from build123d import *

# Parameters (mm, degrees)
F3_DEPTH = 25.4


with BuildPart() as f1:
    # F0 (on Front) → F1 (revolve)
    with BuildSketch(Plane.XZ):
        Polygon((4.520118, 0), (0, 0), (0, -7.362884), (0, -8.120686), (1.567202, -8.120686), (1.567202, -14.471013), (1.567202, -16.159639), (4.721958, -14.471013), (31.757258, 0), (28.579464, 0), (5.046357, -12.607159), (5.046357, 0), align=None)
    revolve(axis=Axis((0, 0, -4.060343), (0, 0, -1)))

    # F2 (on Top) → F3 (cut)
    with BuildSketch(Plane.XY):
        with BuildLine():
            ThreePointArc((-4.51249, 3.106461), (0, 5.478381), (4.51249, 3.106461))
            Line((4.51249, 3.106461), (28.376638, 3.106461))
            ThreePointArc((28.376638, 3.106461), (0, 28.546168), (-28.376638, 3.106461))
            Line((-28.376638, 3.106461), (-4.51249, 3.106461))
        make_face()
        with BuildLine():
            Line((28.376638, -3.106461), (4.51249, -3.106461))
            ThreePointArc((4.51249, -3.106461), (0, -5.478381), (-4.51249, -3.106461))
            Line((-4.51249, -3.106461), (-28.376638, -3.106461))
            ThreePointArc((-28.376638, -3.106461), (0, -28.546168), (28.376638, -3.106461))
        make_face()
    extrude(amount=-F3_DEPTH, mode=Mode.SUBTRACT)


solid = f1.part
Geometry check sheet. Reference: the model listing, model coordinates, mm. A direction names the side the tool comes from. Coordinates: 2 decimals unless noted, no trailing zeros. Order: outer loops, then holes, each group sorted by start corner. A loop starts at its lowest first (then second) coordinate and runs counter-clockwise, first axis right, second up. Notation, with made-up numbers: (-18, -19.5) -> (16, -19.5) arc R32 ccw to (16, 17.5) -> close; hole circle Ø8 at (4, 38). An arc over 180 degrees is marked (long way). Use a Markdown table: item, result. Add a question column.
1. Mould release check, pull along Y, two halves, no side actions. Record for faces 4 (the face through (-0.074, 5.478, -13.209)), 5 (the face through (5.4, -0.6, -12.4)), 6 (the face through (0, 0, 0)): pulls with the +Y half, pulls with the -Y half, needs draft (parallel to the pull), parting line crosses it, or undercut.
2. Cross-section at C-C (x = -0.5). Give the number of separate pieces and of enclosed holes in the cut face, and give its area (3 significant figures).
3. Go/stop test with flat-tipped pins: pin 1 Ø4 at (x, z) = (22, -5) entering from +Y; pin 2 Ø2 at (x, y) = (2.5, 1) entering from -Z; pin 3 Ø4 at (x, z) = (-17.5, -8) entering from -Y; pin 4 Ø1 at (x, y) = (-11.5, -5) entering from -Z. Record where each tip stops, or that it passes through.
4. Set-up check for faces 1 (the face through (0.58, 28.54, -0.86)), 2 (the face through (2.713, -4.255, -6.215)), 3 (the face through (-0.204, -1.554, -12.196)): record each of +Z, -Z, +X, -X, +Y, -Y from which the full face is reachable in a straight line by a thin tool's end or side.
5. Cross-section at B-B (z = -2.75). Enter the section's corners in (x, y).
6. Cross-section at A-A (z = -11.5). Enter the section's corners in (x, y).
7. Material ranges on L1, parallel to Y at x = 0, z = -14; L2, parallel to Y at x = 0, z = -12.25; L3, parallel to X at y = 0.5, z = -5.25, recorded low to high.
Filled sheet:
| question | item | result |
|---|---|---|
| 1 | face 4 | pulls with the +Y half |
| 1 | face 5 | undercut |
| 1 | face 6 | needs draft |
| 2 | separate pieces | 3 |
| 2 | enclosed holes | 0 |
| 2 | area | 139 mm2 |
| 3 | pin 1 | y = 3.11 |
| 3 | pin 2 | z = -16.09 |
| 3 | pin 3 | y = -3.11 |
| 3 | pin 4 | through |
| 4 | face 1 | +Z, -Z |
| 4 | face 2 | +Z |
| 4 | face 3 | -Z |
| 5 | outline | (-26.44, -3.11) -> (-23.24, -3.11) arc R23.45 cw to (-23.24, 3.11) -> (-26.44, 3.11) arc R26.62 ccw to start; circle Ø10.09 at (0, 0); (23.24, -3.11) -> (26.44, -3.11) arc R26.62 ccw to (26.44, 3.11) -> (23.24, 3.11) arc R23.45 cw to start |
| 6 | outline | (-9.79, -3.11) -> (-6.4, -3.11) arc R7.11 cw to (-6.4, 3.11) -> (-9.79, 3.11) arc R10.27 ccw to start; circle Ø10.09 at (0, 0); (6.4, -3.11) -> (9.79, -3.11) arc R10.27 ccw to (9.79, 3.11) -> (6.4, 3.11) arc R7.11 cw to start; hole circle Ø3.13 at (0, 0) |
| 7 | L1 | -5.48 to -1.57, 1.57 to 5.48 |
| 7 | L2 | -5.05 to -1.57, 1.57 to 5.05 |
| 7 | L3 | -21.94 to -18.77, -5.02 to 5.02, 18.77 to 21.94 |
